Can you work these out from the model? Positions are in its coordinate system, mm. Give positions to 0.01 mm unless a question says otherwise; leave off trailing zeros. Loops run counter-clockwise (first coordinate to the right, second up) from the corner with the lowest first, then second, coordinate; pieces in that order, holes last. Notation, with made-up numbers: (66, 52) -> (76, 52) arc R32 cw to (76, 83) -> close; hole circle Ø8 at (14.25, 83). An arc over 180 degrees is marked (long way). One line per question, with ' | ' between items.
from build123d import *

# Parameters (mm, degrees)
CROQUIS1_R              = 3
CROQUIS1_R_2            = 3.4
CROQUIS1_R_3            = 2
CROQUIS1_R_4            = 4.5
CROQUIS1_W              = 12.8
CROQUIS1_H              = 48.5
CROQUIS1_W_2            = 62.75
CROQUIS1_H_2            = 25
CROQUIS1_W_3            = 90.7
CROQUIS1_H_3            = 20
CROQUIS1_W_4            = 81.75
SALIENTE_EXTRUIR1_DEPTH = 4
REDONDEO1_R             = 5


with BuildPart() as part:
    # Croquis1 → Saliente-Extruir1 (new body)
    with BuildSketch(Plane(origin=(0, 0, 0), x_dir=(1, 0, 0), z_dir=(0, 1, 0))):
        with BuildLine():
            Line((0, -35.5), (0, 35.5))
            ThreePointArc((0, 35.5), (1.464466094, 39.035533906), (5, 40.5))
            Line((5, 40.5), (27.5, 40.5))
            Line((27.5, 40.5), (27.5, 70))
            ThreePointArc((27.5, 70), (37.5, 80), (47.5, 70))
            Line((47.5, 70), (47.5, 25))
            ThreePointArc((47.5, 25), (48.964466094, 21.464466094), (52.5, 20))
            Line((52.5, 20), (137.5, 20))
            ThreePointArc((137.5, 20), (141.742640687, 21.757359313), (143.5, 26))
            Line((143.5, 26), (143.5, 26.5))
            ThreePointArc((143.5, 26.5), (145.257359313, 30.742640687), (149.5, 32.5))
            Line((149.5, 32.5), (229.25, 32.5))
            ThreePointArc((229.25, 32.5), (233.492640687, 30.742640687), (235.25, 26.5))
            Line((235.25, 26.5), (235.25, 26))
            ThreePointArc((235.25, 26), (237.007359313, 21.757359313), (241.25, 20))
            Line((241.25, 20), (307.5, 20))
            Line((307.5, 20), (307.5, 42.5))
            ThreePointArc((307.5, 42.5), (308.964466094, 46.035533906), (312.5, 47.5))
            Line((312.5, 47.5), (317, 47.5))
            Line((317, 47.5), (317, 71))
            ThreePointArc((317, 71), (327, 81), (337, 71))
            Line((337, 71), (337, -71))
            ThreePointArc((337, -71), (327, -81), (317, -71))
            Line((317, -71), (317, -47.5))
            Line((317, -47.5), (312.5, -47.5))
            ThreePointArc((312.5, -47.5), (308.964466094, -46.035533906), (307.5, -42.5))
            Line((307.5, -42.5), (307.5, -20))
            Line((307.5, -20), (241.25, -20))
            ThreePointArc((241.25, -20), (237.007359313, -21.757359313), (235.25, -26))
            Line((235.25, -26), (235.25, -26.5))
            ThreePointArc((235.25, -26.5), (233.492640687, -30.742640687), (229.25, -32.5))
            Line((229.25, -32.5), (149.5, -32.5))
            ThreePointArc((149.5, -32.5), (145.257359313, -30.742640687), (143.5, -26.5))
            Line((143.5, -26.5), (143.5, -26))
            ThreePointArc((143.5, -26), (141.742640687, -21.757359313), (137.5, -20))
            Line((137.5, -20), (52.5, -20))
            ThreePointArc((52.5, -20), (48.964466094, -21.464466094), (47.5, -25))
            Line((47.5, -25), (47.5, -70))
            ThreePointArc((47.5, -70), (37.5, -80), (27.5, -70))
            Line((27.5, -70), (27.5, -40.5))
            Line((27.5, -40.5), (5, -40.5))
            ThreePointArc((5, -40.5), (1.464466094, -39.035533906), (0, -35.5))
        make_face()
        with Locations(Location((37.5, 70, 0), (0, 0, 270))):
            Circle(CROQUIS1_R, mode=Mode.SUBTRACT)
        with Locations(Location((144.6, 0, 0), (0, 0, 270))):
            Circle(CROQUIS1_R_2, mode=Mode.SUBTRACT)
        with Locations(Location((153.5, 20.15, 0), (0, 0, 270))):
            Circle(CROQUIS1_R_3, mode=Mode.SUBTRACT)
        with Locations(Location((225.25, 20.15, 0), (0, 0, 270))):
            Circle(CROQUIS1_R_3, mode=Mode.SUBTRACT)
        with Locations(Location((317, 30, 0), (0, 0, 270))):
            Circle(CROQUIS1_R_4, mode=Mode.SUBTRACT)
        with Locations(Location((327, 71, 0), (0, 0, 270))):
            Circle(CROQUIS1_R, mode=Mode.SUBTRACT)
        with Locations(Location((7.5, 30.5, 0), (0, 0, 270))):
            Circle(CROQUIS1_R_4, mode=Mode.SUBTRACT)
        with Locations(Location((327, -71, 0), (0, 0, 90))):
            Circle(CROQUIS1_R, mode=Mode.SUBTRACT)
        with Locations(Location((317, -30, 0), (0, 0, 90))):
            Circle(CROQUIS1_R_4, mode=Mode.SUBTRACT)
        with Locations(Location((225.25, -20.15, 0), (0, 0, 90))):
            Circle(CROQUIS1_R_3, mode=Mode.SUBTRACT)
        with Locations(Location((153.5, -20.15, 0), (0, 0, 90))):
            Circle(CROQUIS1_R_3, mode=Mode.SUBTRACT)
        with Locations(Location((37.5, -70, 0), (0, 0, 90))):
            Circle(CROQUIS1_R, mode=Mode.SUBTRACT)
        with Locations(Location((7.5, -30.5, 0), (0, 0, 90))):
            Circle(CROQUIS1_R_4, mode=Mode.SUBTRACT)
        with Locations((21.9, 0)):
            Rectangle(CROQUIS1_W, CROQUIS1_H, mode=Mode.SUBTRACT)
        with Locations((189.375, 0)):
            Rectangle(CROQUIS1_W_2, CROQUIS1_H_2, mode=Mode.SUBTRACT)
        with Locations((82.4, 0)):
            Rectangle(CROQUIS1_W_3, CROQUIS1_H_3, mode=Mode.SUBTRACT)
        with Locations((286.125, 0)):
            Rectangle(CROQUIS1_W_4, CROQUIS1_H_3, mode=Mode.SUBTRACT)
    extrude(amount=SALIENTE_EXTRUIR1_DEPTH)

    # Redondeo1
    redondeo1_edges = [part.edges().sort_by_distance(p)[0] for p in [
        (127.75, 2, 10),
        (127.75, 2, -10),
        (37.05, 2, -10),
        (37.05, 2, 10),
        (28.3, 2, -24.25),
        (15.5, 2, -24.25),
        (15.5, 2, 24.25),
        (28.3, 2, 24.25),
        (327, 2, 10),
        (327, 2, -10),
        (245.25, 2, -10),
        (245.25, 2, 10),
        (220.75, 2, -12.5),
        (158, 2, -12.5),
        (158, 2, 12.5),
        (220.75, 2, 12.5),
    ]]
    fillet(redondeo1_edges, radius=REDONDEO1_R)


solid = part.part
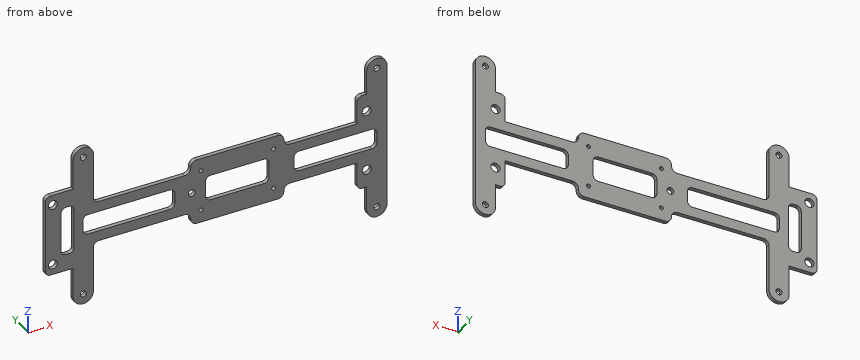
Q1. If we section it at D-D (y = 1.05): State how many separate pieces and enclosed holes the cut face has, plus the area to 3 significant figures.
Entries:
separate pieces: 1 | enclosed holes: 17 | area: 16,100 mm²
Q2. For pin 1 Ø2 at (x, y) = (174.5, 2) entering from -Z; pin 2 Ø1.5 at (x, y) = (92.5, 1.5) entering from +Z; pin 3 Ø2 at (x, y) = (22.5, 3) entering from -Z, each with a flat end and sliding along its axis, tell me the tip position at first contact or that it passes through.
Entries:
pin 1: z = -32.5 | pin 2: z = 20 | pin 3: z = -40.5
Q3. If we section it at B-B (z = -62.5): Write out the boundary of the cut face in (x, y).
Entries:
outline: (27.5, 0) -> (47.5, 0) -> (47.5, 4) -> (27.5, 4) -> close; (317, 0) -> (337, 0) -> (337, 4) -> (317, 4) -> close
Q4. If we section it at A-A (x = 179): Write out the boundary of the cut face in (y, z), plus the area to 3 significant figures.
Entries:
outline: (0, -32.5) -> (4, -32.5) -> (4, -12.5) -> (0, -12.5) -> close; (0, 12.5) -> (4, 12.5) -> (4, 32.5) -> (0, 32.5) -> close | area: 160 mm²
Q5. If we section it at C-C (z = 0): Write out the boundary of the cut face in (x, y).
Entries:
outline: (0, 0) -> (15.5, 0) -> (15.5, 4) -> (0, 4) -> close; (28.3, 0) -> (37.05, 0) -> (37.05, 4) -> (28.3, 4) -> close; (127.75, 0) -> (141.2, 0) -> (141.2, 4) -> (127.75, 4) -> close; (148, 0) -> (158, 0) -> (158, 4) -> (148, 4) -> close; (220.75, 0) -> (245.25, 0) -> (245.25, 4) -> (220.75, 4) -> close; (327, 0) -> (337, 0) -> (337, 4) -> (327, 4) -> close
Q6. If I drill on probe 1 along X at (y, z) = (1.3, 0); probe 2 along Z at (x, y) = (153.5, 1.5); probe 3 along Z at (x, y) = (37, 2.9), over which ranges is the centre line in solid material (lowest first)? Write a range as from..to.
Entries:
probe 1: 0..15.5, 28.3..37.05, 127.75..141.2, 148..158, 220.75..245.25, 327..337 | probe 2: -32.5..-22.15, -18.15..18.15, 22.15..32.5 | probe 3: -79.99..-72.96, -67.04..67.04, 72.96..79.99
